```python
from build123d import *

# Parameters (mm, degrees)
F1_R     = 15
F3_R     = 15
F3_R_2   = 12.5
F4_DEPTH = 20
F5_R     = 13.5
F6_DEPTH = 180


with BuildPart() as f2:
    # F2: sweep along a path in F0
    with BuildLine(Plane.XZ) as f2_path:
        Line((0, 0), (0, 30))
        ThreePointArc((0, 30), (5.8578643763, 44.1421356237), (20, 50))
        Line((20, 50), (200, 50))
    # F1 (on Top) → F2 (sweep)
    with BuildSketch(Plane.XY):
        Circle(F1_R)
    sweep(path=f2_path.line)

    # F3 (on Top) → F4 (cut)
    with BuildSketch(Plane.XY):
        Circle(F3_R)
        Circle(F3_R_2, mode=Mode.SUBTRACT)
    extrude(amount=F4_DEPTH, mode=Mode.SUBTRACT)

    # F5 (on face) → F6 (cut)
    with BuildSketch(Plane.YZ.offset(200)):
        with Locations((0, 50)):
            Circle(F5_R)
    extrude(amount=-F6_DEPTH, mode=Mode.SUBTRACT)


solid = f2.part
```
Verification items for the finished model (mm, model axes). A direction names the side the tool comes from. Coordinates: 2 decimals unless noted, no trailing zeros. Order: outer loops, then holes, each group sorted by start corner. A loop starts at its lowest first (then second) coordinate and runs counter-clockwise, first axis right, second up. Notation, with made-up numbers: (-33.75, 60) -> (-13.75, 60) arc R12 cw to (-13.75, 78) -> close; hole circle Ø3 at (22, -39). An arc over 180 degrees is marked (long way). Answer as CSV lines item,"result". Start each with the question number.
1) Material ranges on L1, parallel to Z at x = 57, y = 0.5; L2, parallel to Y at x = 177, z = 54.5; L3, parallel to Z at x = 85, y = -3, recorded low to high. Write a range as [from, to].
2) Release check for a two-part mould opening along Y. For faces 1 (the face through (111.26, -1.757, 63.385)), 2 (the face through (-14.985, 0.66, 25.07)), 3 (the face through (0, 0, 0)) record: released by +Y, released by -Y, zero draft, split by the parting line, or undercut.
3) Cross-section at B-B, the plane y = 0. Record the boundary of the cut face in (x, z).
4) Set-up check for faces 4 (the face through (-3.4, 12.3, 20)), 5 (the face through (200, -7.85, 38.82)), 6 (the face through (20, 0, 50)): record each of +Z, -Z, +X, -X, +Y, -Y from which the full face is reachable in a straight line by a thin tool's end or side.
5) Cross-section at A-A, the plane x = 80. Record the boundary of the cut face in (y, z).
6) Gauge pin test, flat ends, axial feed: pin 1 Ø4 at (x, y) = (74.5, -3) entering from +Z; pin 2 Ø8 at (x, y) = (157, 5.5) entering from +Z; pin 3 Ø1 at (y, z) = (-10, 18.5) entering from -X; pin 4 Ø15 at (x, y) = (2.5, 2) entering from -Z. Record the tip position at first contact, or that the pin passes through.
7) Cross-section at D-D, the plane z = 26. Record the boundary of the cut face in (x, y).
8) Cross-section at C-C, the plane z = 11.5. Record the boundary of the cut face in (x, y).
Conclusion:
1,L1,"z = [35.01, 36.51], [63.49, 64.99]"
1,L2,"y = [-14.31, -12.73], [12.73, 14.31]"
1,L3,"z = [35.3, 36.84], [63.16, 64.7]"
2,face 1,"undercut"
2,face 2,"split by the parting line"
2,face 3,"zero draft"
3,outline,"(-15, 20) -> (-12.5, 20) -> (-12.5, 0) -> (12.5, 0) -> (12.5, 20) -> (15, 20) -> (15, 30) arc R5 cw to (20, 35) -> (200, 35) -> (200, 36.5) -> (20, 36.5) -> (20, 63.5) -> (200, 63.5) -> (200, 65) -> (20, 65) arc R35 ccw to (-15, 30) -> close"
4,face 4,"-Z"
4,face 5,"+Z, -Z, +X, +Y, -Y"
4,face 6,"+X"
5,outline,"circle Ø30 at (0, 50); hole circle Ø27 at (0, 50)"
6,pin 1,"stops at z = 64.97"
6,pin 2,"stops at z = 64.92"
6,pin 3,"stops at x = -8.12"
6,pin 4,"stops at z = 0"
7,outline,"circle Ø30 at (0, 0)"
8,outline,"circle Ø25 at (0, 0)"
